Part model, mm, in its own coordinate system. Face numbers are marked on the shaded views. A direction names the side the tool comes from. Round coordinates to 2 decimals unless told otherwise and drop trailing zeros. Loops run counter-clockwise (first coordinate to the right, second up) from the corner with the lowest first, then second, coordinate; pieces in that order, holes last. Notation, with made-up numbers: (81.5, 13.5) - (122.5, 13.5) arc R8 cw to (122.5, 26.5) - close; hole circle Ø8 at (88.25, 53.25). An arc over 180 degrees is marked (long way). Put each result on its own line as item: value.
from build123d import *

# Parameters (mm, degrees)
F0_W       = 12.7783659846
F0_H       = 6.3891834579
F0_W_2     = 13.0687858909
F0_H_2     = 7.5508533046
F1_DEPTH   = 25.4
F2_R       = 10.532388255
F3_DEPTH   = 25.4
F4_R       = 2.0535610712
F4_R_2     = 2.1586830731
F4_R_3     = 2.3948426669
F5_DEPTH   = 25.4
F6_R       = 4.2285410778
F6_R_2     = 4.1581451927
F1_FACE2_W = 65.9247562289
F1_FACE2_H = 25.4
F7_DEPTH   = 7.5518533046
F8_R       = 2.677519439
F8_R_2     = 2.6177858958
F9_DEPTH   = 25.4
F10_W      = 11.6166961379
F10_H      = 11.0358633101
F11_DEPTH  = 12.1975312941


with BuildPart() as f1:
    # F0 (on Front) → F1 (new body)
    with BuildSketch(Plane.XZ):
        with Locations((-27.7348635718, 3.194591729)):
            Rectangle(F0_W, F0_H)
        Polygon((-21.3456805795, 6.3891834579), (-21.3456805795, 0), (0, 0), (18.7319237739, 0), (18.7319237739, 7.5508533046), (18.7319237739, 37.7542637289), (6.5343924798, 37.7542637289), (6.5343924798, 28.0633459114), (-8.2768974826, 28.0633459114), (-8.2768974826, 31.655497849), (-11.4714885131, 37.7542637289), (-21.3456805795, 37.7542637289), (-21.3456805795, 14.8112885654), align=None)
        with Locations((25.2663167194, 3.7754266523)):
            Rectangle(F0_W_2, F0_H_2)
    extrude(amount=F1_DEPTH)

    # F2 (on face) → F3 (cut, through all)
    with BuildSketch(Plane.XZ.offset(25.4)):
        with Locations((0, 22.6525589824)):
            Circle(F2_R)
    extrude(amount=-F3_DEPTH, mode=Mode.SUBTRACT)

    # F4 (on face) → F5 (cut, through all)
    with BuildSketch(Plane.XZ.offset(25.4)):
        with Locations((13.2139939815, 22.0717247576)):
            Circle(F4_R)
        with Locations((0, 9.8741920665)):
            Circle(F4_R_2)
        with Locations((-13.2139930502, 22.9429770261)):
            Circle(F4_R_3)
    extrude(amount=-F5_DEPTH, mode=Mode.SUBTRACT)

    # F6 (on face) + F1_face2 (on face) → F7 (cut, through all)
    with BuildSketch(Plane.XY.offset(7.5508533046)):
        with Locations((24.54027161, -12.1975317597)):
            Circle(F6_R)
        with Locations((-27.7348645031, -12.7783669159)):
            Circle(F6_R_2)
    with BuildSketch(Plane(origin=(-1.1616684496, -12.7, 0), x_dir=(1, 0, 0), z_dir=(0, 0, -1))):
        Rectangle(F1_FACE2_W, F1_FACE2_H)
    extrude(amount=-F7_DEPTH, dir=(0, 0, 1), mode=Mode.SUBTRACT)

    # F8 (on face) → F9 (cut, through all)
    with BuildSketch(Plane.XZ.offset(25.4)):
        with Locations((-17.7154634148, 33.833630383)):
            Circle(F8_R)
        with Locations((15.1017084718, 33.6884185672)):
            Circle(F8_R_2)
    extrude(amount=-F9_DEPTH, mode=Mode.SUBTRACT)

    # F10 (on face) → F11 (cut, through all)
    with BuildSketch(Plane.YZ.offset(18.7319237739)):
        with Locations((-12.3427396175, 36.8830133229)):
            Rectangle(F10_W, F10_H)
    extrude(amount=-F11_DEPTH, mode=Mode.SUBTRACT)


solid = f1.part
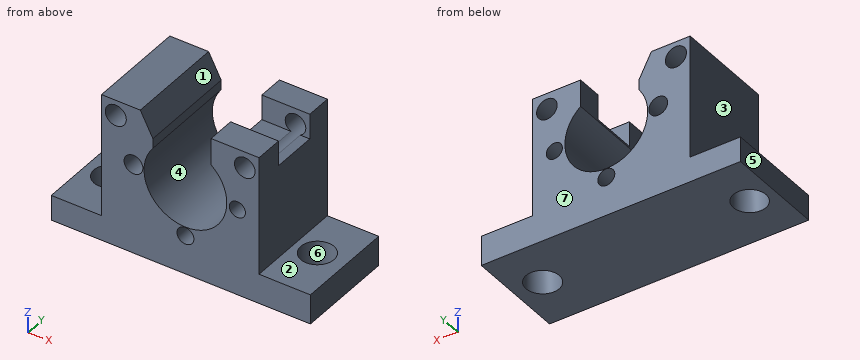
1. Tool access for the marked faces 1, 2 and 3: list every direction of +Z, -Z, +X, -X, +Y, -Y with a clear straight run to the whole face (end or side of a thin tool).
A:
face 1: +Z, +Y, -Y
face 2: +Z, +X, +Y, -Y
face 3: +Z, -X, +Y, -Y
2. Band-saw the part on D-D (y = -20). List the corners of the cut face in (x, z).
A:
outline: (-34.12, 0) - (31.8, 0) - (31.8, 7.55) - (18.73, 7.55) - (18.73, 37.75) - (6.53, 37.75) - (6.53, 30.91) arc R10.53 cw (long way) to (-8.28, 29.17) - (-8.28, 31.66) - (-11.47, 37.75) - (-21.35, 37.75) - (-21.35, 6.39) - (-34.12, 6.39) - close; hole circle Ø5.36 at (-17.72, 33.83); hole circle Ø4.79 at (-13.21, 22.94); hole circle Ø4.32 at (0, 9.87); hole circle Ø4.11 at (13.21, 22.07); hole circle Ø5.24 at (15.1, 33.69)
3. Band-saw the part on A-A (x = 0). List the corners of the cut face in (y, z).
A:
outline: (-25.4, 0) - (0, 0) - (0, 7.72) - (-25.4, 7.72) - close; (-25.4, 12.03) - (0, 12.03) - (0, 12.12) - (-25.4, 12.12) - close
4. Band-saw the part on B-B (y = -14.5). List the corners of the cut face in (x, z).
A:
outline: (-34.12, 0) - (-31.52, 0) - (-31.52, 6.39) - (-34.12, 6.39) - close; (-23.95, 0) - (20.99, 0) - (20.99, 7.55) - (18.73, 7.55) - (18.73, 31.37) - (16.31, 31.37) arc R2.62 cw to (13.9, 31.37) - (6.53, 31.37) - (6.53, 30.91) arc R10.53 cw (long way) to (-8.28, 29.17) - (-8.28, 31.66) - (-11.47, 37.75) - (-21.35, 37.75) - (-21.35, 6.39) - (-23.95, 6.39) - close; (28.09, 0) - (31.8, 0) - (31.8, 7.55) - (28.09, 7.55) - close; hole circle Ø5.36 at (-17.72, 33.83); hole circle Ø4.79 at (-13.21, 22.94); hole circle Ø4.32 at (0, 9.87); hole circle Ø4.11 at (13.21, 22.07)
5. Band-saw the part on C-C (z = 18). List the corners of the cut face in (x, y).
A:
outline: (-21.35, -25.4) - (-9.45, -25.4) - (-9.45, 0) - (-21.35, 0) - close; (9.45, -25.4) - (18.73, -25.4) - (18.73, 0) - (9.45, 0) - close
6. Probe line 1 along X through (y, z) = (-11.75, 22.5); line 2 along X through (y, z) = (-14.5, 26); line 3 along Z through (x, y) = (29.5, -5.25). List the from-to ranges inside material, lowest first. Write a range as [from, to].
A:
line 1: x = [-21.35, -15.57], [-10.86, -10.53], [10.53, 11.21], [15.22, 18.73]
line 2: x = [-21.35, -9.99], [9.99, 18.73]
line 3: z = [0, 7.55]
7. Pin check, flat tips, straight feed: P1, Ø19, axis at x = 0, z = 22.65, coming from the +Y side; P2, Ø1, axis at y = -17.5, z = 23.5, coming from the +X side; P3, Ø5.5, axis at y = -10, z = 34.5, coming from the -X side; P4, Ø1.2, axis at x = 17.5, y = -12.5, coming from the +Z side. Stop position of each tip, or through.
A:
P1: passes through
P2: stops at x = 18.73
P3: stops at x = -21.35
P4: stops at z = 31.37
8. Two-plate mould, pull along X, no slides. Class the marked faces 4, 5, 6 and 7: pulls with the +X half, pulls with the -X half, needs draft (parallel to the pull), parting line crosses it, or undercut.
A:
face 4: undercut
face 5: pulls with the -X half
face 6: undercut
face 7: needs draft
